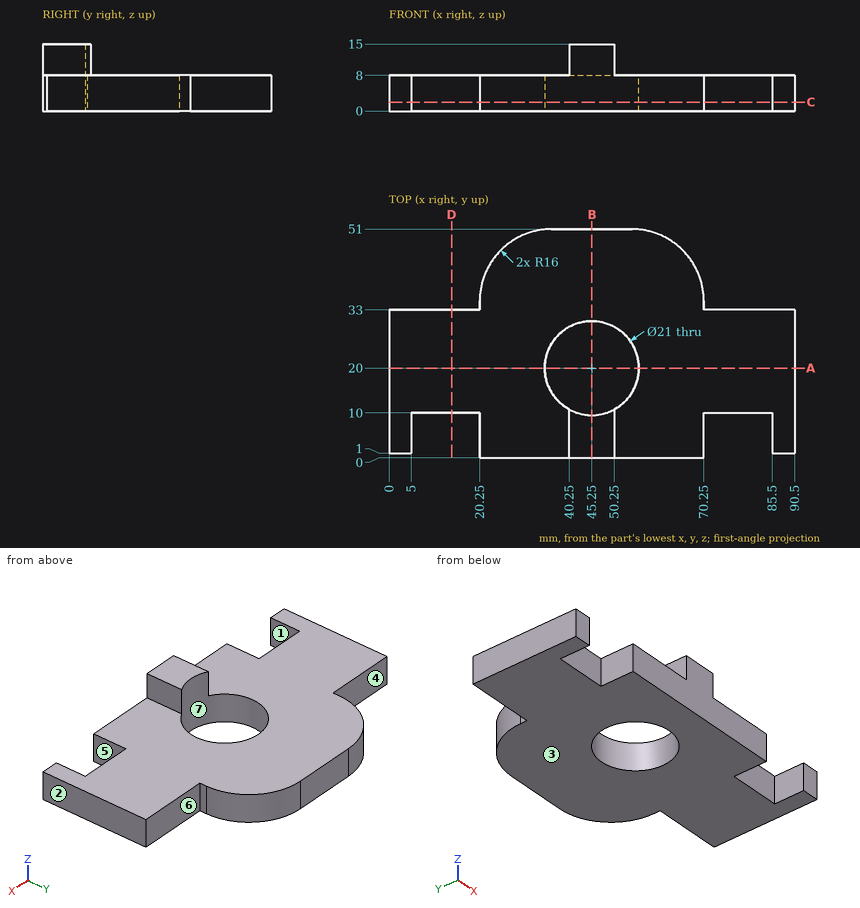
Verification items for this drawing (mm, ordinates from the low corner). A direction names the side the tool comes from. Coordinates: 2 decimals unless noted, no trailing zeros. Write each loop counter-clockwise with the first axis right and the second up, starting at its lowest first coordinate (ties: lowest second). Pieces come first, ordered by that corner, then holes. Notation, with made-up numbers: M -39,66.25 L 16,66.25 A19 cw 16,72.25 Z; hole C -10.5,52 d10. An arc over 180 degrees is marked long. Answer as a JSON object with one key per item and string values. Group by question number.
(1) Gauge pin test, flat ends, axial feed: pin 1 (4 mm diameter, centred on x = 3, z = 4, fed in from -Y); pin 2 (8 mm diameter, centred on y = 44.5, z = 4, fed in from -X) (3 decimals); pin 3 (6.5 mm diameter, centred on x = 75.5, z = 2.5, fed in from +Y). Record the tip position at first contact, or that the pin passes through.
(2) Cross-section at A-A, the plane y = 20. Record the cut outline in (x, z).
(3) Cross-section at D-D, the plane x = 14. Record the cut outline in (y, z), and give its area (3 significant figures).
(4) Release check for a two-part mould opening along X. For the marked faces 1, 2 and 3 record: +X half, -X half, draft (parallel to the pull), parting line (faces both ways), or undercut.
(5) Cross-section at B-B, the plane x = 45.25. Record the cut outline in (y, z).
(6) Material ranges on line 1 (Y direction, x = 45.25, z = 6.75); line 2 (X direction, y = 20, z = 4.5); line 3 (Z direction, x = 64.5, y = 23), recorded low to high.
(7) Cross-section at C-C, the plane z = 2. Record the cut outline in (x, y), and give its area (3 significant figures).
(8) Tool access check on the marked faces 4, 5, 6 and 7. Record the directions out of +Z, -Z, +X, -X, +Y, -Y that give a thin tool (end or side, any length) a straight path to the whole face; none if there is none.
Reply:
{
 "1": {"pin 1": "y = 1", "pin 2": "x = 21.225", "pin 3": "y = 33"},
 "2": {"outline": "M 0,0 L 34.75,0 L 34.75,8 L 0,8 Z; M 55.75,0 L 90.5,0 L 90.5,8 L 55.75,8 Z"},
 "3": {"outline": "M 10,0 L 33,0 L 33,8 L 10,8 Z", "area": "184 mm²"},
 "4": {"face 1": "undercut", "face 2": "+X half", "face 3": "draft"},
 "5": {"outline": "M 0,0 L 9.5,0 L 9.5,15 L 0,15 Z; M 30.5,0 L 51,0 L 51,8 L 30.5,8 Z"},
 "6": {"line 1": "0 to 9.5, 30.5 to 51", "line 2": "0 to 34.75, 55.75 to 90.5", "line 3": "0 to 8"},
 "7": {"outline": "M 0,1 L 5,1 L 5,10 L 20.25,10 L 20.25,0 L 70.25,0 L 70.25,10 L 85.5,10 L 85.5,1 L 90.5,1 L 90.5,33 L 70.25,33 L 70.25,35 A16 ccw 54.25,51 L 36.25,51 A16 ccw 20.25,35 L 20.25,33 L 0,33 Z; hole C 45.25,20 d21", "area": "3,120 mm²"},
 "8": {"face 4": "+Z, -Z, -X, +Y", "face 5": "+Z, -Z, -Y", "face 6": "+Z, -Z, +X, +Y", "face 7": "+Z, -Z"}
}
